CAD build for the part. Positions are in the model's coordinates, mm. Face numbers are marked on the shaded views. A direction names the side the tool comes from. Coordinates: 2 decimals unless noted, no trailing zeros. Order: outer loops, then holes, each group sorted by start corner. A loop starts at its lowest first (then second) coordinate and runs counter-clockwise, first axis right, second up. Notation, with made-up numbers: (81.25, 62.5) - (86.25, 62.5) arc R23 ccw to (86.25, 81.5) - close; hole circle Ø5 at (-4.5, 80.25). An arc over 180 degrees is marked (long way). Use one line per item in the form item = value.
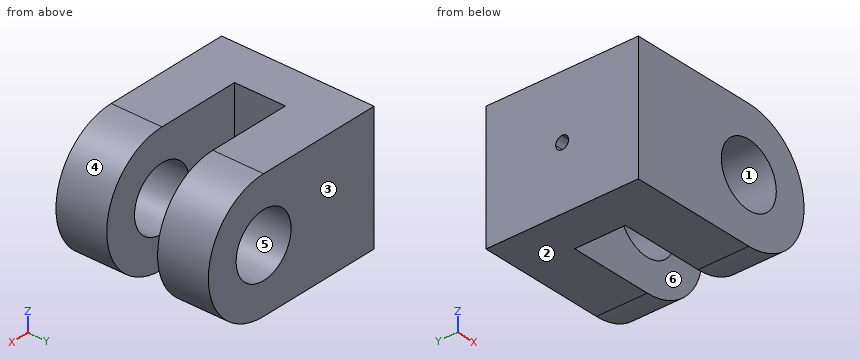
```python
from build123d import *

# Parameters (mm, degrees)
F0_R     = 12.446
F1_DEPTH = 19.9898
F3_R     = 12.446
F4_DEPTH = 19.9898
F5_W     = 17.1654498105
F5_H     = 50.038
F6_DEPTH = 19.9898
F8_DEPTH = 75.058


with BuildPart() as f1:
    # F0 (on Front) → F1 (new body)
    with BuildSketch(Plane.XZ):
        with BuildLine():
            Line((-50.038, -25.019), (0, -25.019))
            ThreePointArc((0, -25.019), (25.019, 0), (0, 25.019))
            Line((0, 25.019), (-50.038, 25.019))
            Line((-50.038, 25.019), (-50.038, -25.019))
        make_face()
        Circle(F0_R, mode=Mode.SUBTRACT)
    extrude(amount=F1_DEPTH)



with BuildPart() as f4:
    # F3 (on offset) → F4 (new body)
    with BuildSketch(Plane.XZ.offset(39.9796)):
        with BuildLine():
            Line((-50.038, 25.019), (-50.038, -25.019))
            Line((-50.038, -25.019), (0, -25.019))
            ThreePointArc((0, -25.019), (25.019, 0), (0, 25.019))
            Line((0, 25.019), (-50.038, 25.019))
        make_face()
        Circle(F3_R, mode=Mode.SUBTRACT)
    extrude(amount=F4_DEPTH)


with BuildPart() as f1_1:
    add(f1.part)

    add(f4.part)  # F6 merges F4
    # F5 (on face) → F6 (join, through all)
    with BuildSketch(Plane.XZ.offset(19.9898)):
        with Locations((-41.4552750947, 0)):
            Rectangle(F5_W, F5_H)
    extrude(amount=F6_DEPTH)

    # F7 (on face) → F8 (cut, through all)
    with BuildSketch(Plane(origin=(-50.038, 0, 0), x_dir=(0, -1, 0), z_dir=(-1, 0, 0))):
        with BuildLine():
            ThreePointArc((29.9847, -2.54), (31.7807512242, -1.7960512242), (32.5247, 0))
            ThreePointArc((32.5247, 0), (31.7807512242, 1.7960512242), (29.9847, 2.54))
            ThreePointArc((29.9847, 2.54), (28.1886487758, 1.7960512242), (27.4447, 0))
            ThreePointArc((27.4447, 0), (28.1886487758, -1.7960512242), (29.9847, -2.54))
        make_face()
    extrude(amount=-F8_DEPTH, mode=Mode.SUBTRACT)


solid = f1_1.part
```
Item 1: Cut at B-B, the plane x = -9. Write the cut outline in (y, z), plus the area to 3 significant figures.
Derived:
outline = (-59.97, -25.02) - (-39.98, -25.02) - (-39.98, -8.6) - (-59.97, -8.6) - close; (-59.97, 8.6) - (-39.98, 8.6) - (-39.98, 25.02) - (-59.97, 25.02) - close; (-19.99, -25.02) - (0, -25.02) - (0, -8.6) - (-19.99, -8.6) - close; (-19.99, 8.6) - (0, 8.6) - (0, 25.02) - (-19.99, 25.02) - close
area = 1,310 mm²
Item 2: Cut at D-D, the plane x = 15. Write the cut outline in (y, z).
Derived:
outline = (-59.97, -20.02) - (-39.98, -20.02) - (-39.98, 20.02) - (-59.97, 20.02) - close; (-19.99, -20.02) - (0, -20.02) - (0, 20.02) - (-19.99, 20.02) - close
Item 3: Cut at A-A, the plane z = 1.5. Write the cut outline in (x, y), plus the area to 3 significant figures.
Derived:
outline = (-50.04, -59.97) - (-12.36, -59.97) - (-12.36, -39.98) - (-32.87, -39.98) - (-32.87, -32.03) - (-50.04, -32.03) - close; (-50.04, -27.93) - (-32.87, -27.93) - (-32.87, -19.99) - (-12.36, -19.99) - (-12.36, 0) - (-50.04, 0) - close; (12.36, -59.97) - (24.97, -59.97) - (24.97, -39.98) - (12.36, -39.98) - close; (12.36, -19.99) - (24.97, -19.99) - (24.97, 0) - (12.36, 0) - close
area = 2,280 mm²
Item 4: 3-axis set-ups, long thin cutter, end or side, ignore diameter. For the marked faces 5 and 6: which of +Z, -Z, +X, -X, +Y, -Y reach the whole face in a straight line?
Derived:
face_5 = +Y, -Y
face_6 = +Z, -Z, +X
Item 5: Cut at C-C, the plane y = -46. Write the cut outline in (x, z).
Derived:
outline = (-50.04, -25.02) - (0, -25.02) arc R25.02 ccw to (0, 25.02) - (-50.04, 25.02) - close; hole circle Ø24.89 at (0, 0)
Item 6: Two-plate mould, pull along Z, no slides. Class the marked faces 1, 2, 3 and 4: +Z half, -Z half, draft (parallel to the pull), parting line (faces both ways), or undercut.
Derived:
face_1 = undercut
face_2 = -Z half
face_3 = draft
face_4 = parting line
Item 7: Drill centre lines: line 1 (Y direction, x = -13, z = 17); line 2 (X direction, y = -29, z = 10); line 3 (X direction, y = -18.5, z = 7.5). Where is each one in solid material? Low to high. Write a range as [from, to].
Derived:
line_1 = [-59.97, -39.98], [-19.99, 0]
line_2 = [-50.04, -32.87]
line_3 = [-50.04, -9.93], [9.93, 23.87]
Item 8: Drop flat-ended pins along their axis: pin 1 (2 mm diameter, centred on y = -50.5, z = -3, fed in from +X); pin 2 (3 mm diameter, centred on y = -8.5, z = 5.5, fed in from +X); pin 3 (22 mm diameter, centred on y = -27, z = 8, fed in from +X). Give the stop position or say it passes through.
Derived:
pin_1 = 24.94
pin_2 = 24.7
pin_3 = 25.02
